The figure shows three views and two pictorial views of one solid part (mm, origin at its lowest corner). Answer the questions. A direction names the side the tool comes from. Coordinates: 2 decimals unless noted, no trailing zeros. Write each loop counter-clockwise with the first axis right and the second up, starting at its lowest first coordinate (ties: lowest second). Pieces come first, ordered by that corner, then holes.
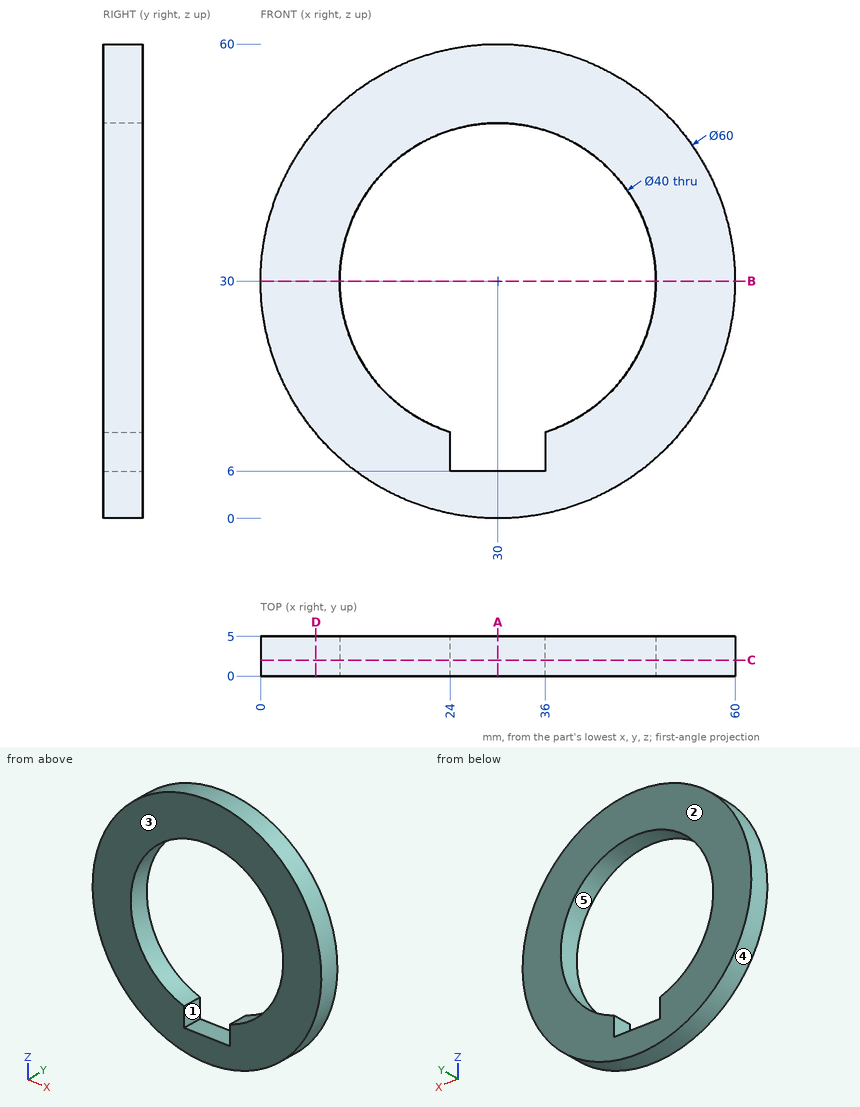
Q1. Determine the mould class of the marked faces 3, 4 and 5 for opening direction X: released by +X, released by -X, zero draft, split by the parting line, or undercut.
Answers below:
face 3: zero draft
face 4: split by the parting line
face 5: undercut
Q2. The part is cut by section D-D, the plane x = 7. Write down the section's boundary in (y, z), then the cut area to 3 significant figures.
Answers below:
outline: (0, 10.74) - (5, 10.74) - (5, 49.26) - (0, 49.26) - close
area: 193 mm2
Q3. The part is cut by section A-A, the plane x = 30. Write down the section's boundary in (y, z), then the cut area to 3 significant figures.
Answers below:
outline: (0, 0) - (5, 0) - (5, 6) - (0, 6) - close; (0, 50) - (5, 50) - (5, 60) - (0, 60) - close
area: 80.0 mm2
Q4. The part is cut by section C-C, the plane y = 2. Write down the section's boundary in (x, z).
Answers below:
outline: circle Ø60 at (30, 30); hole (24, 6) - (36, 6) - (36, 10.92) arc R20 ccw (long way) to (24, 10.92) - close
Q5. The part is cut by section B-B, the plane z = 30. Write down the section's boundary in (x, y), then the cut area to 3 significant figures.
Answers below:
outline: (0, 0) - (10, 0) - (10, 5) - (0, 5) - close; (50, 0) - (60, 0) - (60, 5) - (50, 5) - close
area: 100 mm2
Q6. Given pin 1 (2 mm diameter, centred on x = 12.5, y = 4, fed in from -Z); pin 2 (2 mm diameter, centred on y = 0.5, z = 12, fed in from +X); pin 3 (1.5 mm diameter, centred on y = 4, z = 24.5, fed in from -X), each flat-ended and moving along its own axis, determine where each tip first touches the part or whether it passes through.
Answers below:
pin 1: stops at z = 4.95
pin 2: stops at x = 54.72
pin 3: stops at x = 0.38
Q7. Which of the six approach directions +Z, -Z, +X, -X, +Y, -Y give full straight-line access (tool end or side, diameter ignored) to the marked faces 1 and 2?
Answers below:
face 1: +Y, -Y
face 2: +Z, -Z, +X, -X, +Y
Q8. Find the intervals of material crossed by probe 1 along X at (y, z) = (3.45, 30); probe 2 along X at (y, z) = (2.9, 25.5); probe 3 along Z at (x, y) = (41.5, 2.2), in increasing order.
Answers below:
probe 1: x = 0 to 10, 50 to 60
probe 2: x = 0.34 to 10.51, 49.49 to 59.66
probe 3: z = 2.29 to 13.64, 46.36 to 57.71
